Source: CAD feature listing. Evaluate the final solid. Frame: model axes, mm. A direction names the side the tool comes from. Give positions to 0.01 mm unless a question says otherwise; leave off trailing zeros. Loops run counter-clockwise (first coordinate to the right, second up) from the corner with the lowest first, then second, coordinate; pieces in that order, holes last.
```python
from build123d import *

# Parameters (mm, degrees)
SKETCH_1_W      = 100
SKETCH_1_H      = 70
EXTRUDE_1_DEPTH = 35
SKETCH_3_R      = 34
EXTRUDE_2_DEPTH = 60


with BuildPart() as part:
    # Эскиз1 → Бобышка-Вытянуть1 (new body)
    with BuildSketch(Plane.XY):
        Rectangle(SKETCH_1_W, SKETCH_1_H)
    extrude(amount=EXTRUDE_1_DEPTH)

    # Эскиз3 → Бобышка-Вытянуть2 (add)
    with BuildSketch(Plane(origin=(0, 0, 0), x_dir=(-1, 0, 0), z_dir=(0, 0, -1))):
        with Locations((15, 0)):
            Circle(SKETCH_3_R)
    extrude(amount=-EXTRUDE_2_DEPTH)


solid = part.part
```
(1) Section D-D, the plane y = 27.5. Return the cut outline in (x, z).
A:
outline: (-50, 0) - (50, 0) - (50, 35) - (4.99, 35) - (4.99, 60) - (-34.99, 60) - (-34.99, 35) - (-50, 35) - close
(2) Reachability of faces 4 (the flat face through (22, 0, 35)), 5 (the flat face through (-1, 35, 17)) from +Z, -Z, +X, -X, +Y, -Y: full face, straight path, thin tool, end or side. Return the list, or none.
A:
face 4: +Z
face 5: +Z, -Z, +X, -X, +Y
(3) Section B-B, the plane x = 26. Return the cut outline in (y, z).
A:
outline: (-35, 0) - (35, 0) - (35, 35) - (-35, 35) - close
(4) Section A-A, the plane y = 0. Return the cut outline in (x, z), then the cut area to 3 significant figures.
A:
outline: (-50, 0) - (50, 0) - (50, 35) - (19, 35) - (19, 60) - (-49, 60) - (-49, 35) - (-50, 35) - close
area: 5,200 mm2
(5) First-contact query: pin 1 (8 mm diameter, centred on x = -18, z = 42, fed in from +Y). Flat tip, straight axial feed; report the tip coordinate or a pass-through.
A:
pin 1: stops at y = 34
(6) Mould query, pull axis Y, two halves, no side actions, for faces 1 (the flat face through (-1, -35, 17)), 2 (the flat face through (1, 0, 0)), 3 (the cylindrical face through (10.06, 22.98, 47.32)). Classes: pulls with the +Y half, pulls with the -Y half, needs draft (parallel to the pull), parting line crosses it, or undercut.
A:
face 1: pulls with the -Y half
face 2: needs draft
face 3: parting line crosses it
(7) Ray query, line 1 along Z through (x, y) = (17, -30); line 2 along Y through (x, z) = (-42.5, 56); line 3 along X through (y, z) = (-14.5, 44.5). Return the intervals inside material, ascending.
A:
line 1: z = 0 to 35
line 2: y = -19.99 to 19.99
line 3: x = -45.75 to 15.75
(8) Section C-C, the plane z = 55. Return the cut outline in (x, y), then the cut area to 3 significant figures.
A:
outline: circle Ø68 at (-15, 0)
area: 3,630 mm2
